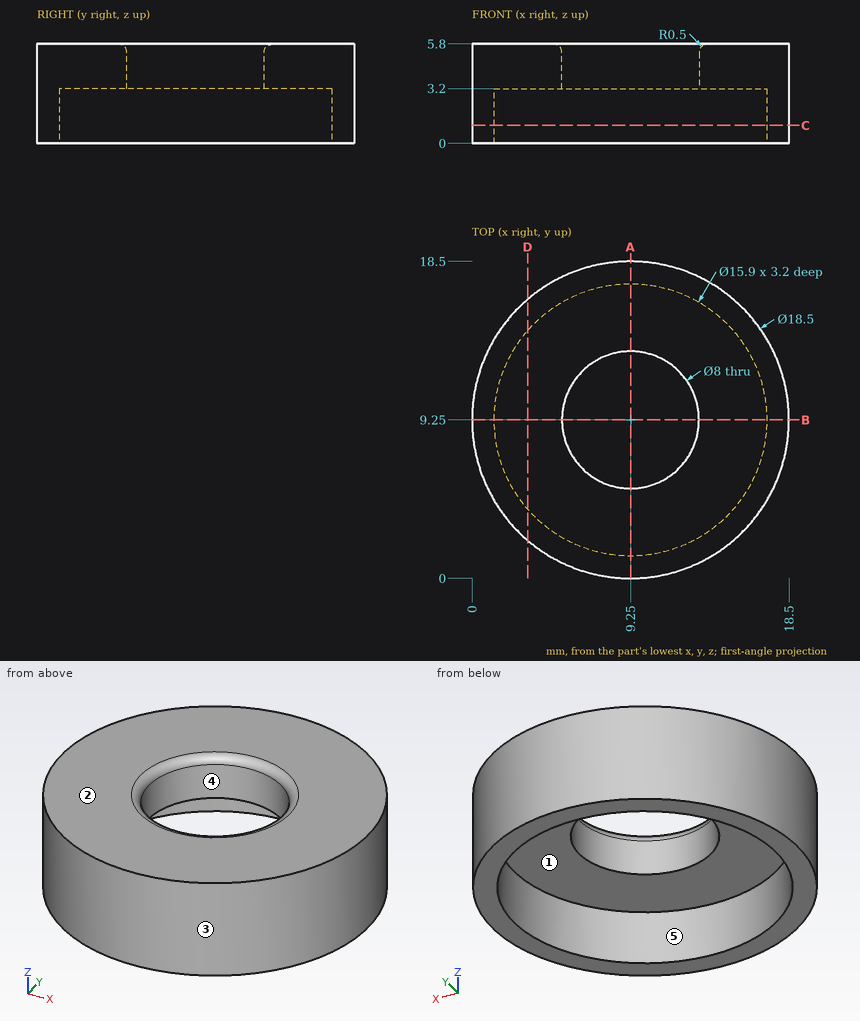
Can you work these out from the drawing? Everything is in mm from the part's minimum corner. A direction names the side the tool comes from. Round coordinates to 2 decimals unless told otherwise and drop trailing zeros. Loops run counter-clockwise (first coordinate to the right, second up) from the corner with the lowest first, then second, coordinate; pieces in that order, holes last. Notation, with made-up numbers: (35, -11) - (65, -11) arc R27 ccw to (65, 18) - close; hole circle Ø5 at (85.5, 18). An arc over 180 degrees is marked (long way). Answer in a Markdown table with one row per item. Add a question column.
Q1. I need wall thicknesses on L1, parallel to Y at x = 9.25, z = 1.65; L2, parallel to X at y = 12.5, z = 1.2; L3, parallel to Z at x = 15.75, y = 10. Which ranges of each line are inside material? Lowest first, please.
Q2. I want a section at D-D on x = 3.25. List the corners of the cut face in (y, z) for me.
Q3. I want a section at C-C on z = 1.05. List the corners of the cut face in (x, y) for me, and give its area (3 significant figures).
Q4. I want a section at A-A on x = 9.25. List the corners of the cut face in (y, z) for me.
Q5. We'd pull the mould along Y, two halves only. Please class the marked faces 1, 2 and 3: pulls with the +Y half, pulls with the -Y half, needs draft (parallel to the pull), parting line crosses it, or undercut.
Q6. Which directions (+Z, -Z, +X, -X, +Y, -Y) give clear straight access to the entire face, cutting with the end or side of a thin tool? Please do the marked faces 4 and 5.
Q7. For pin 1 Ø5 at (x, y) = (9.25, 9.25) entering from +Z; pin 2 Ø1 at (y, z) = (16, 3.5) entering from -X, each with a flat end and sliding along its axis, tell me the tip position at first contact or that it passes through.
A:
| question | item | result |
|---|---|---|
| 1 | L1 | 0 to 1.3, 17.2 to 18.5 |
| 1 | L2 | 0.59 to 1.99, 16.51 to 17.91 |
| 1 | L3 | 3.2 to 5.8 |
| 2 | outline | (2.21, 0) - (4.03, 0) - (4.03, 3.2) - (14.47, 3.2) - (14.47, 0) - (16.29, 0) - (16.29, 5.8) - (2.21, 5.8) - close |
| 3 | outline | circle Ø18.5 at (9.25, 9.25); hole circle Ø15.9 at (9.25, 9.25) |
| 3 | area | 70.2 mm^2 |
| 4 | outline | (0, 0) - (1.3, 0) - (1.3, 3.2) - (5.25, 3.2) - (5.25, 5.3) arc R0.5 ccw to (4.75, 5.8) - (0, 5.8) - close; (13.25, 3.2) - (17.2, 3.2) - (17.2, 0) - (18.5, 0) - (18.5, 5.8) - (13.75, 5.8) arc R0.5 ccw to (13.25, 5.3) - close |
| 5 | face 1 | undercut |
| 5 | face 2 | needs draft |
| 5 | face 3 | parting line crosses it |
| 6 | face 4 | +Z, -Z |
| 6 | face 5 | -Z |
| 7 | pin 1 | through |
| 7 | pin 2 | x = 2.43 |
